from build123d import *

# Parameters (mm, degrees)
CROQUIS1_W                 = 34
CROQUIS1_H                 = 22
CROQUIS1_R                 = 5.1
SALIENTE_EXTRUIR1_DEPTH    = 15
CORTAR_EXTRUIR1_DEPTH      = 5.2
CORTAR_EXTRUIR2_DEPTH      = 5.2
CORTAR_EXTRUIR3_DEPTH      = 4
CORTAR_EXTRUIR3_DEPTH_BACK = 4
CROQUIS5_R                 = 3.1
CORTAR_EXTRUIR4_DEPTH      = 4
CORTAR_EXTRUIR5_START      = -4
CROQUIS6_R                 = 3.1
CORTAR_EXTRUIR5_DEPTH      = 4
REDONDEO1_R                = 5


with BuildPart() as part:
    # Croquis1 → Saliente-Extruir1 (new body)
    with BuildSketch(Plane(origin=(0, 0, 0), x_dir=(1, 0, 0), z_dir=(0, 1, 0))):
        with Locations((17, 11)):
            Rectangle(CROQUIS1_W, CROQUIS1_H)
        with Locations(Location((17, 11, 0), (0, 0, 270))):
            Circle(CROQUIS1_R, mode=Mode.SUBTRACT)
    extrude(amount=SALIENTE_EXTRUIR1_DEPTH)

    # Croquis2 → Cortar-Extruir1 (cut)
    with BuildSketch(Plane.ZY.offset(-2)):
        Polygon((-16.1, 10.444486373), (-16.1, 15), (-5.9, 15), (-5.9, 10.444486373), (-5.9, 4.555513627), (-11, 1.611027254), (-16.1, 4.555513627), align=None)
    extrude(amount=-CORTAR_EXTRUIR1_DEPTH, mode=Mode.SUBTRACT)

    # Croquis3 → Cortar-Extruir2 (cut)
    with BuildSketch(Plane(origin=(32, 0, 0), x_dir=(0, 0, -1), z_dir=(1, 0, 0))):
        Polygon((5.9, 15), (5.9, 4.555513627), (11, 1.611027254), (16.1, 4.555513627), (16.1, 15), align=None)
    extrude(amount=-CORTAR_EXTRUIR2_DEPTH, mode=Mode.SUBTRACT)

    # Croquis4 → Cortar-Extruir3 (cut, two sides: drawn at the far end of the back side and taken through both)
    with BuildSketch(Plane(origin=(0, 7.5, 0), x_dir=(1, 0, 0), z_dir=(0, 1, 0)).offset(-CORTAR_EXTRUIR3_DEPTH_BACK)):
        Polygon((8.5, 6.092522712), (17, 1.185045424), (25.5, 6.092522712), (25.5, 15.907477288), (17, 20.814954576), (8.5, 15.907477288), align=None)
    extrude(amount=CORTAR_EXTRUIR3_DEPTH + CORTAR_EXTRUIR3_DEPTH_BACK, mode=Mode.SUBTRACT)

    # Croquis5 → Cortar-Extruir4 (cut)
    with BuildSketch(Plane(origin=(34, 0, 0), x_dir=(0, 0, -1), z_dir=(1, 0, 0))):
        with Locations((11, 7.5)):
            Circle(CROQUIS5_R)
    extrude(amount=-CORTAR_EXTRUIR4_DEPTH, mode=Mode.SUBTRACT)

    # Croquis6 → Cortar-Extruir5 (cut)
    with BuildSketch(Plane.ZY.offset(CORTAR_EXTRUIR5_START)):
        with Locations(Location((-11, 7.5, 0), (0, 0, 180))):
            Circle(CROQUIS6_R)
    extrude(amount=CORTAR_EXTRUIR5_DEPTH, mode=Mode.SUBTRACT)

    # Redondeo1
    redondeo1_edges = [part.edges().sort_by_distance(p)[0] for p in [
        (17, 15, -22),
        (17, 0, -22),
        (17, 0, 0),
        (17, 15, 0),
    ]]
    fillet(redondeo1_edges, radius=REDONDEO1_R)


solid = part.part
Input: part model. Units: mm. Frame: model coordinates. A direction names the side the tool comes from. Coordinates: 2 decimals unless noted, no trailing zeros. Order: outer loops, then holes, each group sorted by start corner. A loop starts at its lowest first (then second) coordinate and runs counter-clockwise, first axis right, second up. Notation, with made-up numbers: M -21.75,65 L 22.25,65 A23 cw 22.25,100 Z; hole C 54,14.5 d6. An arc over 180 degrees is marked long. Answer in a Markdown table with one row per item.
(1) Section query D-D, the plane x = 20.5. Output: boundary loops of the cut face in (y, z), plus the area to 3 significant figures.
Numbers:
| item | result |
|---|---|
| outline | M 0,-17 A5 ccw 5,-22 L 10,-22 A5 ccw 15,-17 L 15,-14.71 L 11.5,-14.71 L 11.5,-18.79 L 3.5,-18.79 L 3.5,-14.71 L 0,-14.71 Z; M 0,-7.29 L 3.5,-7.29 L 3.5,-3.21 L 11.5,-3.21 L 11.5,-7.29 L 15,-7.29 L 15,-5 A5 ccw 10,0 L 5,0 A5 ccw 0,-5 Z |
| area | 132 mm^2 |
(2) Section query C-C, the plane z = -14.5. Output: boundary loops of the cut face in (x, y).
Numbers:
| item | result |
|---|---|
| outline | M 0,0 L 13.29,0 L 13.29,3.5 L 8.5,3.5 L 8.5,11.5 L 13.29,11.5 L 13.29,15 L 7.2,15 L 7.2,3.63 L 2,3.63 L 2,15 L 0,15 Z; M 20.71,0 L 34,0 L 34,15 L 32,15 L 32,3.63 L 26.8,3.63 L 26.8,15 L 20.71,15 L 20.71,11.5 L 25.5,11.5 L 25.5,3.5 L 20.71,3.5 Z |
(3) Section query B-B, the plane y = 7.5. Output: boundary loops of the cut face in (x, z), plus the area to 3 significant figures.
Numbers:
| item | result |
|---|---|
| outline | M 0,-22 L 34,-22 L 34,-14.1 L 32,-14.1 L 32,-16.1 L 26.8,-16.1 L 26.8,-5.9 L 32,-5.9 L 32,-7.9 L 34,-7.9 L 34,0 L 0,0 L 0,-7.9 L 2,-7.9 L 2,-5.9 L 7.2,-5.9 L 7.2,-16.1 L 2,-16.1 L 2,-14.1 L 0,-14.1 Z; hole M 8.5,-15.91 L 17,-20.81 L 25.5,-15.91 L 25.5,-6.09 L 17,-1.19 L 8.5,-6.09 Z |
| area | 367 mm^2 |
(4) Draft query along Z for faces 5 (the flat face through (0, 6, -8)), 6 (the cylindrical face through (17, 1, -20)), 7 (the flat face through (29, 10, -16.1)). Return one class per face: pulls with the +Z half, pulls with the -Z half, needs draft (parallel to the pull), parting line crosses it, or undercut.
Numbers:
| item | result |
|---|---|
| face 5 | needs draft |
| face 6 | pulls with the -Z half |
| face 7 | undercut |
(5) Material intervals for line 1 (X direction, y = 9.25, z = -6.75); line 2 (X direction, y = 12.9, z = -11); line 3 (Y direction, x = 23.5, z = -12.75), sorted ascending. Write a range as [from, to].
Numbers:
| item | result |
|---|---|
| line 1 | x = [0, 2], [7.2, 8.5], [25.5, 26.8], [32, 34] |
| line 2 | x = [0, 2], [7.2, 11.9], [22.1, 26.8], [32, 34] |
| line 3 | y = [0, 3.5], [11.5, 15] |
(6) Contact query for flat-ended pins moving along their axis: pin 1 Ø3.5 at (y, z) = (7.5, -11) entering from +X; pin 2 Ø3 at (x, z) = (14, -19) entering from -Y; pin 3 Ø1 at (x, y) = (22.5, 11) entering from -Z; pin 4 Ø8 at (x, z) = (17, -11) entering from -Y. Output: stop coordinate, or through.
Numbers:
| item | result |
|---|---|
| pin 1 | stops at x = 26.8 |
| pin 2 | stops at y = 0.03 |
| pin 3 | stops at z = -21.97 |
| pin 4 | passes through |
(7) Access query for faces 1 (the cylindrical face through (33.01, 9.6, -8.72)), 2 (the flat face through (4.56, 3.06, -13.51)), 3 (the flat face through (21.19, 7.444, -3.604)), 4 (the cylindrical face through (1, 7.4, -7.9)). Directions: +Z, -Z, +X, -X, +Y, -Y. A direction counts if a zero-diameter tool reaches every point of the face in a straight line with its end or side. Return the directions, or none.
Numbers:
| item | result |
|---|---|
| face 1 | +X |
| face 2 | +Y |
| face 3 | none |
| face 4 | -X |
(8) Section query A-A, the plane x = 29.5. Output: boundary loops of the cut face in (y, z).
Numbers:
| item | result |
|---|---|
| outline | M 0,-17 A5 ccw 5,-22 L 10,-22 A5 ccw 15,-17 L 15,-16.1 L 4.56,-16.1 L 1.61,-11 L 4.56,-5.9 L 15,-5.9 L 15,-5 A5 ccw 10,0 L 5,0 A5 ccw 0,-5 Z |
